Could you check a few things on this model? Use its own coordinates, in mm. Coordinates: 2 decimals unless noted, no trailing zeros. Loops run counter-clockwise (first coordinate to the right, second up) from the corner with the lowest first, then second, coordinate; pieces in that order, holes last. Notation, with made-up numbers: (31.25, 57) -> (90.25, 57) arc R14 cw to (90.25, 68) -> close; hole circle Ø5 at (77.5, 49.5). An arc over 180 degrees is marked (long way). One line per question, with ' | ' between items.
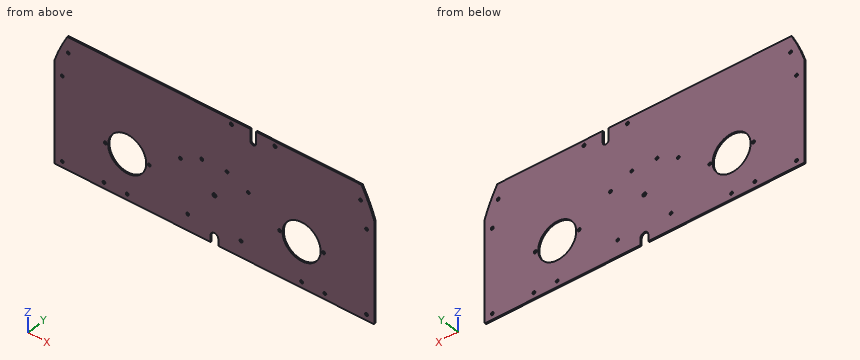
```python
from build123d import *

# Parameters (mm, degrees)
BOSS_EXTRU_1_DEPTH       = 1.5
ESQUISSE7_R              = 1.5
ENL_V_MAT_EXTRU_5_DEPTH  = 230.841793415
ESQUISSE8_R              = 19.627416998
ESQUISSE8_R_2            = 1.5
ENL_V_MAT_EXTRU_6_DEPTH  = 230.841793415
ESQUISSE9_R              = 1.5
ESQUISSE9_R_2            = 2
ENL_V_MAT_EXTRU_7_DEPTH  = 230.841793415
ENL_V_MAT_EXTRU_8_DEPTH  = 230.841793415
CONG_1_R                 = 1
ESQUISSE11_R             = 1.5
ENL_V_MAT_EXTRU_9_DEPTH  = 230.841793415
ESQUISSE12_R             = 1.6
ESQUISSE12_W             = 330
ESQUISSE12_H             = 75
ENL_V_MAT_EXTRU_10_DEPTH = 230.841793415


with BuildPart() as part:
    # Esquisse1 → Boss.-Extru.1 (new body)
    with BuildSketch(Plane(origin=(0, 0, 0), x_dir=(1, 0, 0), z_dir=(0, 1, 0))):
        with BuildLine():
            Line((0, 49), (165, 49))
            Line((165, 49), (165, -55.235857919))
            ThreePointArc((165, -55.235857919), (127.908511428, -117.963607542), (68.381283989, -160))
            Line((68.381283989, -160), (0, -160))
            Line((0, -160), (0, 49))
        make_face()
    extrude(amount=BOSS_EXTRU_1_DEPTH)

    # Symétrie1: part across plane


with BuildPart() as part_1:
    add(part.part)
    add(part.part.mirror(Plane(origin=(0, 1.5, -49), x_dir=(0, 0, 1), z_dir=(1, 0, 0))))

    # Esquisse7 → Enlèv. mat.-Extru.5 (cut, through all)
    with BuildSketch(Plane(origin=(0, 1.5, 0), x_dir=(1, 0, 0), z_dir=(0, 1, 0))):
        with Locations(Location((-157, -43, 0), (0, 0, 270))):
            Circle(ESQUISSE7_R)
        with Locations(Location((157, -43, 0), (0, 0, 270))):
            Circle(ESQUISSE7_R)
        with Locations(Location((157, 43, 0), (0, 0, 270))):
            Circle(ESQUISSE7_R)
        with Locations(Location((-157, 43, 0), (0, 0, 270))):
            Circle(ESQUISSE7_R)
        with Locations(Location((-114, 43, 0), (0, 0, 270))):
            Circle(ESQUISSE7_R)
        with Locations(Location((-90, 43, 0), (0, 0, 270))):
            Circle(ESQUISSE7_R)
        with Locations(Location((90, 43, 0), (0, 0, 90))):
            Circle(ESQUISSE7_R)
        with Locations(Location((114, 43, 0), (0, 0, 90))):
            Circle(ESQUISSE7_R)
    extrude(amount=-ENL_V_MAT_EXTRU_5_DEPTH, mode=Mode.SUBTRACT)

    # Esquisse8 → Enlèv. mat.-Extru.6 (cut, through all)
    with BuildSketch(Plane(origin=(0, 1.5, 0), x_dir=(1, 0, 0), z_dir=(0, 1, 0))):
        with Locations(Location((-90, 2.5, 0), (0, 0, 270))):
            Circle(ESQUISSE8_R)
        with Locations(Location((-112.627416998, 2.5, 0), (0, 0, 270))):
            Circle(ESQUISSE8_R_2)
        with Locations(Location((-67.372583002, 2.5, 0), (0, 0, 270))):
            Circle(ESQUISSE8_R_2)
        with Locations(Location((112.627416998, 2.5, 0), (0, 0, 90))):
            Circle(ESQUISSE8_R_2)
        with Locations(Location((67.372583002, 2.5, 0), (0, 0, 90))):
            Circle(ESQUISSE8_R_2)
        with Locations(Location((90, 2.5, 0), (0, 0, 90))):
            Circle(ESQUISSE8_R)
    extrude(amount=-ENL_V_MAT_EXTRU_6_DEPTH, mode=Mode.SUBTRACT)

    # Esquisse9 → Enlèv. mat.-Extru.7 (cut, through all)
    with BuildSketch(Plane(origin=(0, 1.5, 0), x_dir=(1, 0, 0), z_dir=(0, 1, 0))):
        with Locations(Location((27.5, 32.5, 0), (0, 0, 270))):
            Circle(ESQUISSE9_R)
        with Locations(Location((-13, -30, 0), (0, 0, 270))):
            Circle(ESQUISSE9_R)
        with Locations(Location((35, -20, 0), (0, 0, 270))):
            Circle(ESQUISSE9_R)
        with Locations(Location((-27.5, 32.5, 0), (0, 0, 90))):
            Circle(ESQUISSE9_R)
        with Locations(Location((0, 0, 0), (0, 0, 270))):
            Circle(ESQUISSE9_R_2)
        with Locations(Location((-35, -20, 0), (0, 0, 90))):
            Circle(ESQUISSE9_R)
        with Locations(Location((13, -30, 0), (0, 0, 90))):
            Circle(ESQUISSE9_R)
        with BuildLine():
            Line((4, 49), (4, 42))
            ThreePointArc((4, 42), (0, 38), (-4, 42))
            Line((-4, 42), (-4, 49))
            ThreePointArc((-4, 49), (0, 53), (4, 49))
        make_face()
    extrude(amount=-ENL_V_MAT_EXTRU_7_DEPTH, mode=Mode.SUBTRACT)

    # Esquisse10 → Enlèv. mat.-Extru.8 (cut, through all)
    with BuildSketch(Plane(origin=(0, 1.5, 0), x_dir=(1, 0, 0), z_dir=(0, 1, 0))):
        with BuildLine():
            Line((43, -73), (43, -150))
            ThreePointArc((43, -150), (40, -153), (37, -150))
            Line((37, -150), (37, -73))
            ThreePointArc((37, -73), (40, -70), (43, -73))
        make_face()
    extrude(amount=-ENL_V_MAT_EXTRU_8_DEPTH, mode=Mode.SUBTRACT)

    # Congé1
    cong_1_edges = [part_1.edges().sort_by_distance(p)[0] for p in [
        (-165, 0.75, -49),
        (165, 0.75, -49),
    ]]
    fillet(cong_1_edges, radius=CONG_1_R)

    # Esquisse11 → Enlèv. mat.-Extru.9 (cut, through all)
    with BuildSketch(Plane(origin=(0, 1.5, 0), x_dir=(1, 0, 0), z_dir=(0, 1, 0))):
        with Locations(Location((-150.869773386, -69.240966765, 0), (0, 0, 270))):
            Circle(ESQUISSE11_R)
        with Locations(Location((-116.399964779, -118.351375994, 0), (0, 0, 270))):
            Circle(ESQUISSE11_R)
        with Locations(Location((-66.72330927, -152, 0), (0, 0, 270))):
            Circle(ESQUISSE11_R)
        with Locations(Location((66.72330927, -152, 0), (0, 0, 90))):
            Circle(ESQUISSE11_R)
        with Locations(Location((116.399964779, -118.351375994, 0), (0, 0, 90))):
            Circle(ESQUISSE11_R)
        with Locations(Location((150.869773386, -69.240966765, 0), (0, 0, 90))):
            Circle(ESQUISSE11_R)
        with Locations(Location((-15, -152, 0), (0, 0, 270))):
            Circle(ESQUISSE11_R)
        with Locations(Location((15, -152, 0), (0, 0, 90))):
            Circle(ESQUISSE11_R)
    extrude(amount=-ENL_V_MAT_EXTRU_9_DEPTH, mode=Mode.SUBTRACT)

    # Esquisse12 → Enlèv. mat.-Extru.10 (cut, through all)
    with BuildSketch(Plane(origin=(0, 1.5, 0), x_dir=(1, 0, 0), z_dir=(0, 1, 0))):
        with Locations(Location((17.5, -80, 0), (0, 0, 270))):
            Circle(ESQUISSE12_R)
        with Locations(Location((62.5, -80, 0), (0, 0, 270))):
            Circle(ESQUISSE12_R)
        with Locations((0, -122.5)):
            Rectangle(ESQUISSE12_W, ESQUISSE12_H)
    extrude(amount=-ENL_V_MAT_EXTRU_10_DEPTH, mode=Mode.SUBTRACT)


solid = part_1.part
```
Q1. Imagine slicing it at B-B on y = 0.35. Give the number of separate pieces and of enclosed holes in the cut face, plus the area to 3 significant figures.
Values follow:
separate pieces: 1 | enclosed holes: 25 | area: 41,100 mm2
Q2. For pin 1 (2.5 mm diameter, centred on x = -112.63, z = -2.5, fed in from -Y), with a flat end and sliding along its axis, tell me the tip position at first contact or that it passes through.
Values follow:
pin 1: passes through
Q3. Imagine slicing it at A-A on z = 9.5. Write out the boundary of the cut face in (x, y), plus the area to 3 significant figures.
Values follow:
outline: (-165, 0) -> (-105.53, 0) -> (-105.53, 1.5) -> (-165, 1.5) -> close; (-74.47, 0) -> (74.47, 0) -> (74.47, 1.5) -> (-74.47, 1.5) -> close; (105.53, 0) -> (165, 0) -> (165, 1.5) -> (105.53, 1.5) -> close | area: 402 mm2
Q4. Please list where these lines run through material, in increasing order: L1, parallel to X at y = 1.1, z = -32.5; L2, parallel to X at y = 0.95, z = 43; L3, parallel to Z at x = -157, y = 0.7. Write a range as [from, to].
Values follow:
L1: x = [-165, -29], [-26, 26], [29, 165] | L2: x = [-165, -158.5], [-155.5, 155.5], [158.5, 165] | L3: z = [-49, -44.5], [-41.5, 41.5], [44.5, 75.01]
